Geometry check sheet. Reference: the model listing, model coordinates, mm. A direction names the side the tool comes from. Coordinates: 2 decimals unless noted, no trailing zeros. Write each loop counter-clockwise with the first axis right and the second up, starting at its lowest first coordinate (ties: lowest second). Pieces come first, ordered by that corner, then holes.
from build123d import *

# Parameters (mm, degrees)
BOSS_EXTRUDE1_DEPTH = 0.92
FILLET3_R           = 0.2
BOSS_EXTRUDE2_DEPTH = 2.7
FILLET4_R           = 0.1


with BuildPart() as part:
    # Sketch2 → Boss-Extrude1 (new body)
    with BuildSketch(Plane(origin=(0, 0, 0), x_dir=(1, 0, 0), z_dir=(0, 1, 0))):
        with BuildLine():
            Line((8.774632583, 14.872725815), (15.174632583, 14.872725815))
            ThreePointArc((15.174632583, 14.872725815), (17.324632583, 12.722725815), (15.174632583, 10.572725815))
            Line((15.174632583, 10.572725815), (8.774632583, 10.572725815))
            ThreePointArc((8.774632583, 10.572725815), (6.624632583, 12.722725815), (8.774632583, 14.872725815))
        make_face()
    extrude(amount=BOSS_EXTRUDE1_DEPTH)

    # Fillet3
    fillet3_edges = [part.edges().sort_by_distance(p)[0] for p in [
        (17.324632583, 0.92, -12.722725815),
        (11.974632583, 0.92, -14.872725815),
        (6.624632583, 0.92, -12.722725815),
        (11.974632583, 0.92, -10.572725815),
    ]]
    fillet(fillet3_edges, radius=FILLET3_R)

    # Sketch5 → Boss-Extrude2 (add)
    with BuildSketch(Plane(origin=(0, 0.92, 0), x_dir=(1, 0, 0), z_dir=(0, 1, 0))):
        with BuildLine():
            Line((8.774632583, 14.672725815), (15.174632583, 14.672725815))
            ThreePointArc((15.174632583, 14.672725815), (17.124632583, 12.722725815), (15.174632583, 10.772725815))
            Line((15.174632583, 10.772725815), (8.774632583, 10.772725815))
            ThreePointArc((8.774632583, 10.772725815), (6.824632583, 12.722725815), (8.774632583, 14.672725815))
        make_face()
    extrude(amount=BOSS_EXTRUDE2_DEPTH)

    # Fillet4
    fillet4_edges = [part.edges().sort_by_distance(p)[0] for p in [
        (6.824632583, 3.62, -12.722725815),
        (11.974632583, 3.62, -10.772725815),
        (17.124632583, 3.62, -12.722725815),
        (11.974632583, 3.62, -14.672725815),
    ]]
    fillet(fillet4_edges, radius=FILLET4_R)


solid = part.part
1. Sectioned sample at C-C, the plane y = 2.5. Record the boundary of the cut face in (x, z).
Computed values:
outline: (8.77, -14.67) - (15.17, -14.67) arc R1.95 ccw to (15.17, -10.77) - (8.77, -10.77) arc R1.95 ccw to start
2. Access from +Z, -Z, +X, -X, +Y, -Y to the whole of each face (thin tool, end or side, straight path). Record for faces 1 (the flat face through (12, 2, -14.673)), 2 (the cylindrical face through (6.825, 2.202, -12.68)), 3 (the cylindrical face through (17.124, 2.202, -12.766)), 4 (the flat face through (12, 2, -10.773)).
Computed values:
face 1: -Z, +X, -X, +Y
face 2: -X, +Y
face 3: +X, +Y
face 4: +Z, +X, -X, +Y
3. Sectioned sample at A-A, the plane x = 13.5. Record the boundary of the cut face in (y, z), and give its area (3 significant figures).
Computed values:
outline: (0, -14.87) - (0.72, -14.87) arc R0.2 ccw to (0.92, -14.67) - (3.52, -14.67) arc R0.1 ccw to (3.62, -14.57) - (3.62, -10.87) arc R0.1 ccw to (3.52, -10.77) - (0.92, -10.77) arc R0.2 ccw to (0.72, -10.57) - (0, -10.57) - close
area: 14.5 mm2
4. Sectioned sample at B-B, the plane y = 0.4. Record the boundary of the cut face in (x, z).
Computed values:
outline: (8.77, -14.87) - (15.17, -14.87) arc R2.15 ccw to (15.17, -10.57) - (8.77, -10.57) arc R2.15 ccw to start
5. Gauge pin test, flat ends, axial feed: pin 1 Ø2 at (x, y) = (12, 2.5) entering from +Z; pin 2 Ø2 at (x, y) = (10, 3) entering from -Z; pin 3 Ø1.5 at (y, z) = (2.5, -14) entering from -X. Record the tip position at first contact, or that the pin passes through.
Computed values:
pin 1: stops at z = -10.77
pin 2: stops at z = -14.67
pin 3: stops at x = 6.9
6. Thickness scan on line 1 along Z through (x, y) = (13.25, 3.35); line 2 along X through (y, z) = (1.4, -12.75); line 3 along X through (y, z) = (0.6, -11.15). Record the ranges inside material, lowest first.
Computed values:
line 1: z = -14.67 to -10.77
line 2: x = 6.82 to 17.12
line 3: x = 7.31 to 16.64
